```python
from build123d import *

# Parameters (mm, degrees)
F0_W      = 66.8829083443
F0_H      = 130.1987469196
F1_DEPTH  = 7.7312737703
F2_R      = 1.27
F3_W      = 65.0993585587
F3_H      = 100.7702499628
F1_FACE_W = 64.3429083443
F1_FACE_H = 127.6587469196
F4_DEPTH  = 2.286
F5_W      = 64.9341493845
F5_H      = 100.1578532159
F6_DEPTH  = 7.62
F7_W      = 64.3429083443
F7_H      = 15.6222133744
F8_DEPTH  = 2.54
F9_W      = 33.9078493416
F9_H      = 3.507707268
F9_R      = 1.2895427644
F9_R_2    = 1.8868222833
F10_DEPTH = 2.54
F11_DEPTH = 2.54
F12_W     = 64.3429083443
F12_H     = 11.8786803293
F13_DEPTH = 2.54
F14_W     = 11.2873837352
F14_H     = 10.0332312286
F15_DEPTH = 2.54
F16_R     = 1.27
F17_W     = 8.7473837352
F17_H     = 7.4932312286
F18_DEPTH = 1.27
F19_R     = 1.8325750533
F20_DEPTH = 10.16
F21_W     = 9.5073804259
F21_H     = 1.0563768446
F22_DEPTH = 5.08
F23_W     = 1.6090744175
F23_H     = 20.8489261568
F23_W_2   = 1.8709015567
F23_H_2   = 8.5872001946
F24_DEPTH = 1.27


with BuildPart() as f1:
    # F0 (on Front) → F1 (new body)
    with BuildSketch(Plane.XZ):
        Rectangle(F0_W, F0_H)
    extrude(amount=F1_DEPTH)

    # F2
    f2_edges = [f1.edges().sort_by_distance(p)[0] for p in [
        (0, -7.731274, -65.099373),
        (33.441454, -7.731274, 0),
        (0, -7.731274, 65.099373),
        (-33.441454, -7.731274, 0),
        (0, 0, -65.099373),
        (33.441454, 0, 0),
        (0, 0, 65.099373),
        (-33.441454, 0, 0),
        (-33.441454, -3.865637, 65.099373),
        (33.441454, -3.865637, -65.099373),
        (33.441454, -3.865637, 65.099373),
        (-33.441454, -3.865637, -65.099373),
    ]]
    fillet(f2_edges, radius=F2_R)

    # F3 (on Front) + F1_face (on face) → F4 (cut)
    with BuildSketch(Plane.XZ):
        with Locations((0, -7.4506e-06)):
            Rectangle(F3_W, F3_H)
    with BuildSketch(Plane.XZ.offset(7.7312737703)):
        Rectangle(F1_FACE_W, F1_FACE_H)
    extrude(amount=-F4_DEPTH, mode=Mode.SUBTRACT)

    # F5 (on Front) → F6 (join)
    with BuildSketch(Plane.XZ):
        with Locations((0.0237450004, -1.8717665225)):
            Rectangle(F5_W, F5_H)
    extrude(amount=F6_DEPTH)

    # F7 (on face) → F8 (join)
    with BuildSketch(Plane.XZ.offset(5.4452737703)):
        with Locations((0, 56.0182667726)):
            Rectangle(F7_W, F7_H)
    extrude(amount=F8_DEPTH)

    # F9 (on face) → F10 (cut)
    with BuildSketch(Plane.XZ.offset(7.9852737703)):
        with Locations((0.5013104528, 59.1038409621)):
            Rectangle(F9_W, F9_H)
        with Locations((-22.5284751505, 59.5681518316)):
            Circle(F9_R)
        with Locations((21.9313502312, 59.2368096113)):
            Circle(F9_R_2)
    extrude(amount=-F10_DEPTH, mode=Mode.SUBTRACT)

    # F9 (on face) → F11 (cut)
    with BuildSketch(Plane.XZ.offset(7.9852737703)):
        with Locations((0.5013104528, 59.1038409621)):
            Rectangle(F9_W, F9_H)
        with Locations((-22.5284751505, 59.5681518316)):
            Circle(F9_R)
        with Locations((21.9313502312, 59.2368096113)):
            Circle(F9_R_2)
    extrude(amount=-F11_DEPTH, mode=Mode.SUBTRACT)

    # F12 (on face) → F13 (join)
    with BuildSketch(Plane.XZ.offset(5.4452737703)):
        with Locations((0, -57.8900332952)):
            Rectangle(F12_W, F12_H)
    extrude(amount=F13_DEPTH)

    # F14 (on face) → F15 (join)
    with BuildSketch(Plane.XZ):
        with Locations((21.7194668949, 54.1001018137)):
            Rectangle(F14_W, F14_H)
    extrude(amount=-F15_DEPTH)

    # F16
    f16_edges = [f1.edges().sort_by_distance(p)[0] for p in [
        (27.363159, 2.54, 54.100102),
        (21.719467, 2.54, 59.116717),
        (16.075775, 2.54, 54.100102),
        (21.719467, 2.54, 49.083486),
    ]]
    fillet(f16_edges, radius=F16_R)

    # F17 (on face) → F18 (cut)
    with BuildSketch(Plane(origin=(0, 2.54, 0), x_dir=(-1, 0, 0), z_dir=(0, 1, 0))):
        with Locations((-21.7194668949, 54.1001018137)):
            Rectangle(F17_W, F17_H)
    extrude(amount=-F18_DEPTH, mode=Mode.SUBTRACT)

    # F19 (on face) → F20 (cut)
    with BuildSketch(Plane(origin=(0, 0, -65.0993734598), x_dir=(1, 0, 0), z_dir=(0, 0, -1))):
        with Locations((-22.2030133009, 3.3965744078)):
            Circle(F19_R)
    extrude(amount=-F20_DEPTH, mode=Mode.SUBTRACT)

    # F21 (on face) → F22 (cut)
    with BuildSketch(Plane(origin=(0, 0, -65.0993734598), x_dir=(1, 0, 0), z_dir=(0, 0, -1))):
        with Locations((-7.6575875282, 3.9393249899)):
            Rectangle(F21_W, F21_H)
    extrude(amount=-F22_DEPTH, mode=Mode.SUBTRACT)

    # F23 (on face) → F24 (join)
    with BuildSketch(Plane.YZ.offset(33.4414541721)):
        with Locations((-4.0922162589, 31.9034513086)):
            Rectangle(F23_W, F23_H)
        with Locations((-3.992605838, -18.6585467309)):
            Rectangle(F23_W_2, F23_H_2)
    extrude(amount=F24_DEPTH)


solid = f1.part
```
Build history of the part. All positions in model axes, mm. A direction names the side the tool comes from. Give positions to 0.01 mm unless a question says otherwise; leave off trailing zeros. Loops run counter-clockwise (first coordinate to the right, second up) from the corner with the lowest first, then second, coordinate; pieces in that order, holes last. Notation, with made-up numbers: (36.5, -1) -> (48.5, -1) arc R27 ccw to (48.5, 26) -> close; hole circle Ø3 at (16, 62.5). An arc over 180 degrees is marked (long way). One line per question, with ' | ' between items.
Q1. Cut at D-D, the plane x = -8.5. Write the cut outline in (y, z).
Filled sheet:
outline: (-7.99, -63.83) -> (-7.73, -63.83) arc R1.27 ccw to (-6.46, -65.1) -> (-4.47, -65.1) -> (-4.47, -60.02) -> (-3.41, -60.02) -> (-3.41, -65.1) -> (-1.27, -65.1) arc R1.27 ccw to (0, -63.83) -> (0, 63.83) arc R1.27 ccw to (-1.27, 65.1) -> (-6.46, 65.1) arc R1.27 ccw to (-7.73, 63.83) -> (-7.99, 63.83) -> (-7.99, 60.86) -> (-5.45, 60.86) -> (-5.45, 57.35) -> (-7.99, 57.35) -> (-7.99, 48.21) -> (-7.62, 48.21) -> (-7.62, -51.95) -> (-7.99, -51.95) -> close
Q2. Drop flat-ended pins along their axis: pin 1 (0.6 mm diameter, centred on x = 34, y = -3.5, fed in from +Z); pin 2 (4 mm diameter, centred on x = 5, z = 36.5, fed in from +Y); pin 3 (1.4 mm diameter, centred on x = 34.5, y = -4, fed in from -Z). Give the stop position or say it passes through.
Filled sheet:
pin 1: stops at z = 42.33 | pin 2: stops at y = 0 | pin 3: stops at z = -22.95
Q3. Pull direction Z, two halves, no side cores. Call faces 1 (the flat face through (0, -4, 65.099)), 2 (the cylindrical face through (-21.3, -6.73, 59.96)), 3 (the flat face through (0, -7.985, -58)): pulls with the +Z half, pulls with the -Z half, needs draft (parallel to the pull), parting line crosses it, or undercut.
Filled sheet:
face 1: pulls with the +Z half | face 2: undercut | face 3: needs draft
Q4. Drill centre lines: line 1 along Z through (x, y) = (-7, -6); line 2 along X through (y, z) = (-3, 29); line 3 along Y through (x, z) = (6.5, 6.5). Where is each one in solid material? Low to high. Write a range as [from, to].
Filled sheet:
line 1: z = [-65.1, 57.35], [60.86, 65.1] | line 2: x = [-33.44, 33.44] | line 3: y = [-7.62, 0]
Q5. Tool access for faces 4 (the cylindrical face through (21.5, -6.7, 57.4)), 5 (the flat face through (22, 1.27, 54)), 6 (the flat face through (-8, -3.411, -63)): list every direction of +Z, -Z, +X, -X, +Y, -Y with a clear straight run to the whole face (end or side of a thin tool).
Filled sheet:
face 4: -Y | face 5: +Y | face 6: -Z
Q6. Cut at B-B, the plane x = 0. Write the cut outline in (y, z), plus the area to 3 significant figures.
Filled sheet:
outline: (-7.99, -63.83) -> (-7.73, -63.83) arc R1.27 ccw to (-6.46, -65.1) -> (-1.27, -65.1) arc R1.27 ccw to (0, -63.83) -> (0, 63.83) arc R1.27 ccw to (-1.27, 65.1) -> (-6.46, 65.1) arc R1.27 ccw to (-7.73, 63.83) -> (-7.99, 63.83) -> (-7.99, 60.86) -> (-5.45, 60.86) -> (-5.45, 57.35) -> (-7.99, 57.35) -> (-7.99, 48.21) -> (-7.62, 48.21) -> (-7.62, -51.95) -> (-7.99, -51.95) -> close | area: 992 mm²
